Input: part model. Units: mm. Frame: model coordinates. Face numbers are marked on the shaded views. A direction names the side the tool comes from. Coordinates: 2 decimals unless noted, no trailing zeros. Loops run counter-clockwise (first coordinate to the right, second up) from the corner with the lowest first, then second, coordinate; pieces in that order, holes last. Notation, with made-up numbers: M 67.25,-17.75 L 89.25,-17.75 A21 ccw 89.25,-5.75 Z; hole C -22,74 d10. An arc over 180 degrees is marked long. Use a Markdown table: item, result. Add a question column.
1. Line query: L1, parallel to Y at x = -9.5, z = -2.5; L2, parallel to Y at x = -9, z = 14; L3, parallel to Y at x = 0, z = 2.75. Output: solid intervals per line, ascending. Write a range as [from, to].
2. Set-up query: the marked faces 1, 2 and 3. Return all of +Z, -Z, +X, -X, +Y, -Y with unobstructed straight access to the full face (end or side cutting, diameter ignored); none if empty.
3. Section D-D on y = -11. Output: boundary loops of the cut face in (x, z), then the cut area to 3 significant figures.
4. Pin query (flat end, axial travel): pin 1 (17.5 mm diameter, centred on x = -2, z = -7.5, fed in from +Y); pin 2 (5 mm diameter, centred on x = -17, y = -3.5, fed in from +Z); pin 3 (8 mm diameter, centred on x = -8, z = 7.5, fed in from -Y); pin 4 (5 mm diameter, centred on x = -7.5, y = 27, fed in from +Z). Return the tip coordinate at first contact, or that it passes through.
5. Section B-B on x = -8.5. Output: boundary loops of the cut face in (y, z).
6. Section A-A on y = 15. Output: boundary loops of the cut face in (x, z), then the cut area to 3 significant figures.
```python
from build123d import *

# Parameters (mm, degrees)
F0_R      = 22
F0_R_2    = 19
F0_R_3    = 16
F0_R_4    = 13
F0_R_5    = 10
F0_R_6    = 7
F0_R_7    = 4
F1_DEPTH  = 15
F2_DEPTH  = 20
F3_DEPTH  = 24
F4_DEPTH  = 28
F5_DEPTH  = 31
F6_DEPTH  = 34
F7_DEPTH  = 40
F8_SIZE   = 4
F9_R      = 17.5
F10_DEPTH = 3
F11_R     = 11.5
F12_DEPTH = 2
F13_R     = 4.8
F14_DEPTH = 30
F15_R     = 1.5
F16_DEPTH = 12.5


# Not quite as in the source:
# - a feature names something its author has since deleted; it is built from what else it names


with BuildPart() as f1:
    # F0 (on Front) → F1 (new body)
    with BuildSketch(Plane.XZ):
        Circle(F0_R)
        Circle(F0_R_2, mode=Mode.SUBTRACT)
        Circle(F0_R_2)
        Circle(F0_R_3, mode=Mode.SUBTRACT)
        Circle(F0_R_3)
        Circle(F0_R_4, mode=Mode.SUBTRACT)
        Circle(F0_R_4)
        Circle(F0_R_5, mode=Mode.SUBTRACT)
        Circle(F0_R_5)
        Circle(F0_R_6, mode=Mode.SUBTRACT)
        Circle(F0_R_6)
        Circle(F0_R_7, mode=Mode.SUBTRACT)
        Circle(F0_R_7)
    extrude(amount=F1_DEPTH)

    # F0 (on Front) → F2 (join)
    with BuildSketch(Plane.XZ):
        Circle(F0_R_2)
        Circle(F0_R_3, mode=Mode.SUBTRACT)
        Circle(F0_R_3)
        Circle(F0_R_4, mode=Mode.SUBTRACT)
        Circle(F0_R_4)
        Circle(F0_R_5, mode=Mode.SUBTRACT)
        Circle(F0_R_5)
        Circle(F0_R_6, mode=Mode.SUBTRACT)
        Circle(F0_R_6)
        Circle(F0_R_7, mode=Mode.SUBTRACT)
        Circle(F0_R_7)
    extrude(amount=F2_DEPTH)

    # F0 (on Front) → F3 (join)
    with BuildSketch(Plane.XZ):
        Circle(F0_R_3)
        Circle(F0_R_4, mode=Mode.SUBTRACT)
        Circle(F0_R_4)
        Circle(F0_R_5, mode=Mode.SUBTRACT)
        Circle(F0_R_5)
        Circle(F0_R_6, mode=Mode.SUBTRACT)
        Circle(F0_R_6)
        Circle(F0_R_7, mode=Mode.SUBTRACT)
        Circle(F0_R_7)
    extrude(amount=F3_DEPTH)

    # F0 (on Front) → F4 (join)
    with BuildSketch(Plane.XZ):
        Circle(F0_R_4)
        Circle(F0_R_5, mode=Mode.SUBTRACT)
        Circle(F0_R_5)
        Circle(F0_R_6, mode=Mode.SUBTRACT)
        Circle(F0_R_6)
        Circle(F0_R_7, mode=Mode.SUBTRACT)
        Circle(F0_R_7)
    extrude(amount=F4_DEPTH)

    # F0 (on Front) → F5 (join)
    with BuildSketch(Plane.XZ):
        Circle(F0_R_5)
        Circle(F0_R_6, mode=Mode.SUBTRACT)
        Circle(F0_R_6)
        Circle(F0_R_7, mode=Mode.SUBTRACT)
        Circle(F0_R_7)
    extrude(amount=F5_DEPTH)

    # F0 (on Front) → F6 (join)
    with BuildSketch(Plane.XZ):
        Circle(F0_R_6)
        Circle(F0_R_7, mode=Mode.SUBTRACT)
        Circle(F0_R_7)
    extrude(amount=F6_DEPTH)

    # F0 (on Front) → F7 (join)
    with BuildSketch(Plane.XZ):
        Circle(F0_R_7)
    extrude(amount=F7_DEPTH)

    # F8
    f8_edges = [f1.edges().sort_by_distance(p)[0] for p in [
        (-4, -40, 0),
    ]]
    chamfer(f8_edges, length=F8_SIZE)

    # F9 (on face) → F10 (join)
    with BuildSketch(Plane(origin=(0, 0, 0), x_dir=(-1, 0, 0), z_dir=(0, 1, 0))):
        Circle(F9_R)
    extrude(amount=F10_DEPTH)

    # F11 (on face) → F12 (join)
    with BuildSketch(Plane(origin=(0, 3, 0), x_dir=(-1, 0, 0), z_dir=(0, 1, 0))):
        Circle(F11_R)
    extrude(amount=F12_DEPTH)

    # F13 (on face) → F14 (join)
    with BuildSketch(Plane(origin=(0, 5, 0), x_dir=(-1, 0, 0), z_dir=(0, 1, 0))):
        Circle(F13_R)
    extrude(amount=F14_DEPTH)

    # F15 (on Top) → F16 (cut, symmetric)
    with BuildSketch(Plane.XY):
        with Locations((0, 15)):
            Circle(F15_R)
    extrude(amount=F16_DEPTH, both=True, mode=Mode.SUBTRACT)


solid = f1.part
```
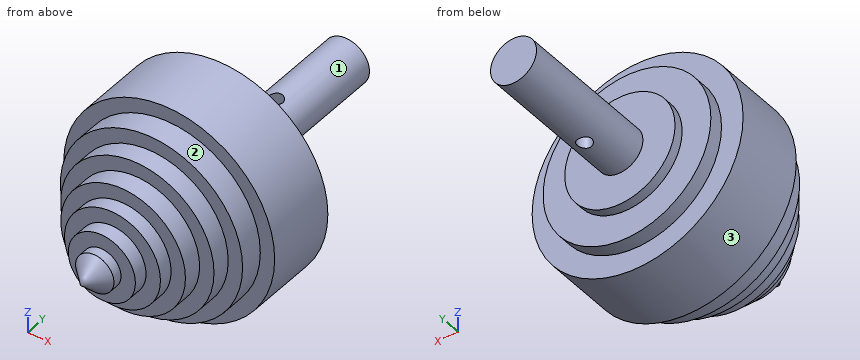
Answers below:
| question | item | result |
|---|---|---|
| 1 | L1 | y = [-31, 5] |
| 1 | L2 | y = [-20, 3] |
| 1 | L3 | y = [-37.25, 13.5], [16.5, 35] |
| 2 | face 1 | +Y |
| 2 | face 2 | -Y |
| 2 | face 3 | +Y, -Y |
| 3 | outline | C 0,0 d44 |
| 3 | area | 1,520 mm² |
| 4 | pin 1 | stops at y = 35 |
| 4 | pin 2 | stops at z = 16.55 |
| 4 | pin 3 | stops at y = -34 |
| 4 | pin 4 | passes through |
| 5 | outline | M -31,-5.27 L -28,-5.27 L -28,-9.84 L -24,-9.84 L -24,-13.56 L -20,-13.56 L -20,-16.99 L -15,-16.99 L -15,-20.29 L 0,-20.29 L 0,-15.3 L 3,-15.3 L 3,-7.75 L 5,-7.75 L 5,7.75 L 3,7.75 L 3,15.3 L 0,15.3 L 0,20.29 L -15,20.29 L -15,16.99 L -20,16.99 L -20,13.56 L -24,13.56 L -24,9.84 L -28,9.84 L -28,5.27 L -31,5.27 Z |
| 6 | outline | M -1.5,-4.56 L -1.5,4.56 A4.8 ccw Z; M 1.5,-4.56 A4.8 ccw 1.5,4.56 Z |
| 6 | area | 44.1 mm² |
